from build123d import *

# Parameters (mm, degrees)
F1_DEPTH = 86.868
F2_R     = 0.654509
F4_DEPTH = 63.246


with BuildPart() as f1:
    # F0 (on Front) → F1 (new body, symmetric)
    with BuildSketch(Plane.XZ):
        with BuildLine():
            ThreePointArc((37.085507, 26.82781), (22.84608, 7.465189), (0, 0))
            Line((0, 0), (29.826211, 0))
            Line((29.826211, 0), (29.826211, -8.521775))
            Line((29.826211, -8.521775), (37.085507, 26.82781))
        make_face()
    extrude(amount=F1_DEPTH, both=True)

    # F2
    f2_edges = [f1.edges().sort_by_distance(p)[0] for p in [
        (37.085507, 0, 26.82781),
        (29.826211, 0, -8.521775),
    ]]
    fillet(f2_edges, radius=F2_R)

    # F3 (on Right) → F4 (cut)
    with BuildSketch(Plane.YZ):
        Polygon((-90.376258, -20.586515), (-65.263629, 54.75137), (-99.720493, 31.098777), align=None)
        Polygon((99.720493, 31.098777), (65.263629, 54.75137), (90.376258, -20.586515), align=None)
    extrude(amount=F4_DEPTH, mode=Mode.SUBTRACT)


solid = f1.part
The model under review builds one solid part; all positions refer to its coordinate system, in mm. A direction names the side the tool comes from. Round coordinates to 2 decimals unless told otherwise and drop trailing zeros. Loops run counter-clockwise (first coordinate to the right, second up) from the corner with the lowest first, then second, coordinate; pieces in that order, holes last. Notation, with made-up numbers: (87.25, -26.5) - (131.25, -26.5) arc R22 cw to (131.25, 10.5) - close; hole circle Ø7 at (-21.5, -32.75). An arc over 180 degrees is marked (long way). Use CSV: the item, a comma, the result in double quotes.
(1) Machinability: for faces 1 (the flat face through (25.775, -81.328, 6.559)), 2 (the flat face through (15, -1, 0)), which of the approach directions +Z, -Z, +X, -X, +Y, -Y give a long, thin tool a straight path to every point of the face, cutting with its end or side? Answer none if there is none.
Working result:
face 1,"+Z, +X, -X, -Y"
face 2,"-Z, -X, +Y, -Y"
(2) Take a section at C-C, the plane z = 3.5. Give the boundary of the cut face in (x, y), plus the area to 3 significant figures.
Working result:
outline,"(16.01, -82.35) - (32.29, -82.35) - (32.29, 82.35) - (16.01, 82.35) - close"
area,"2,680 mm^2"
(3) Take a section at A-A, the plane y = -7.5. Give the boundary of the cut face in (x, z), plus the area to 3 significant figures.
Working result:
outline,"(0, 0) - (29.83, 0) - (29.83, -2.08) arc R0.65 ccw to (31.12, -2.21) - (35.79, 20.52) arc R0.65 ccw to (34.57, 20.96) arc R39.34 cw to start"
area,"196 mm^2"
(4) Take a section at B-B, the plane x = 12. Give the boundary of the cut face in (y, z), plus the area to 3 significant figures.
Working result:
outline,"(-83.51, 0) - (83.51, 0) - (82.87, 1.94) - (-82.87, 1.94) - close"
area,"323 mm^2"
(5) Clearance check with flat-ended pins moving along their axes: P1, Ø0.6, axis at y = 13.5, z = -1.5, coming from the -X side; P2, Ø10, axis at y = 57, z = 16.5, coming from the +X side; P3, Ø6, axis at x = 19, z = 7.5, coming from the +Y side; P4, Ø2, axis at x = 16.5, z = 3.5, coming from the +Y side. State where each tip first meets the part, or that it passes through.
Working result:
P1,"stops at x = 29.83"
P2,"stops at x = 35.8"
P3,"stops at y = 82.01"
P4,"stops at y = 82.68"
(6) For line 1 (Z direction, x = 28, y = 34.5); line 2 (X direction, y = 45, z = -0.75); line 3 (X direction, y = -9.5, z = 6), list the stretches that pass through material, from the lowest coordinate up.
Working result:
line 1,"z = 0 to 11.92"
line 2,"x = 29.83 to 31.42"
line 3,"x = 20.67 to 32.81"
